```python
from build123d import *

# Parameters (mm, degrees)
CROQUIS1_R              = 1.7
SALIENTE_EXTRUIR1_DEPTH = 2
SALIENTE_EXTRUIR2_DEPTH = 6.5
MATRIZL1_COUNT          = 6
MATRIZL1_PITCH          = 2


with BuildPart() as part:
    # Croquis1 → Saliente-Extruir1 (new body)
    with BuildSketch(Plane(origin=(0, 0, 0), x_dir=(1, 0, 0), z_dir=(0, 1, 0))):
        with BuildLine():
            Line((-8, 6), (8, 6))
            Line((8, 6), (8, 3.665719575))
            ThreePointArc((8, 3.665719575), (8.133788189, 2.858848044), (8.520833333, 2.138336419))
            ThreePointArc((8.520833333, 2.138336419), (9.25, 0), (8.520833333, -2.138336419))
            ThreePointArc((8.520833333, -2.138336419), (8.133788189, -2.858848044), (8, -3.665719575))
            Line((8, -3.665719575), (8, -6))
            Line((8, -6), (-8, -6))
            Line((-8, -6), (-8, -3.665719575))
            ThreePointArc((-8, -3.665719575), (-8.133788189, -2.858848044), (-8.520833333, -2.138336419))
            ThreePointArc((-8.520833333, -2.138336419), (-9.25, 0), (-8.520833333, 2.138336419))
            ThreePointArc((-8.520833333, 2.138336419), (-8.133788189, 2.858848044), (-8, 3.665719575))
            Line((-8, 3.665719575), (-8, 6))
        make_face()
        with Locations((5.75, 0)):
            Circle(CROQUIS1_R, mode=Mode.SUBTRACT)
        with Locations((-5.75, 0)):
            Circle(CROQUIS1_R, mode=Mode.SUBTRACT)
    extrude(amount=SALIENTE_EXTRUIR1_DEPTH)

    # Croquis4 → Saliente-Extruir2 (add)
    with BuildSketch(Plane(origin=(3.25, 0, 0), x_dir=(0, 0, -1), z_dir=(1, 0, 0))):
        Polygon((-6, 2), (-4, 2), (-4.9, 2.9), (-5.1, 2.9), align=None)
    saliente_extruir2 = extrude(amount=-SALIENTE_EXTRUIR2_DEPTH)

    # MatrizL1: Saliente-Extruir2 ×6
    with Locations(*[(0, 0, -i * MATRIZL1_PITCH) for i in range(1, MATRIZL1_COUNT)]):
        add(saliente_extruir2)


solid = part.part
```
Input: part model. Units: mm. Frame: model coordinates. A direction names the side the tool comes from. Give positions to 0.01 mm unless a question says otherwise; leave off trailing zeros. Order: outer loops, then holes, each group sorted by start corner. A loop starts at its lowest first (then second) coordinate and runs counter-clockwise, first axis right, second up.
1. Cut plane D-D (x = -1). Return loops of the section in (y, z).
Computed:
outline: (0, -6) - (2, -6) - (2.9, -5.1) - (2.9, -4.9) - (2, -4) - (2.9, -3.1) - (2.9, -2.9) - (2, -2) - (2.9, -1.1) - (2.9, -0.9) - (2, 0) - (2.9, 0.9) - (2.9, 1.1) - (2, 2) - (2.9, 2.9) - (2.9, 3.1) - (2, 4) - (2.9, 4.9) - (2.9, 5.1) - (2, 6) - (0, 6) - close
2. Cut plane A-A (y = 1.8). Return loops of the section in (x, z).
Computed:
outline: (-8.52, -2.14) arc R2.5 cw to (-8, -3.67) - (-8, -6) - (8, -6) - (8, -3.67) arc R2.5 cw to (8.52, -2.14) arc R3.5 ccw to (8.52, 2.14) arc R2.5 cw to (8, 3.67) - (8, 6) - (-8, 6) - (-8, 3.67) arc R2.5 cw to (-8.52, 2.14) arc R3.5 ccw to start; hole circle Ø3.4 at (-5.75, 0); hole circle Ø3.4 at (5.75, 0)
3. Pin query (flat end, axial travel): pin 1 Ø3 at (x, z) = (-6, 2) entering from +Y; pin 2 Ø1 at (y, z) = (0.5, -4.5) entering from +X; pin 3 Ø2.5 at (x, z) = (5.75, 0) entering from -Y; pin 4 Ø0.7 at (y, z) = (2.5, -0.5) entering from -X. Return the tip coordinate at first contact, or that it passes through.
Computed:
pin 1: stops at y = 2
pin 2: stops at x = 8
pin 3: passes through
pin 4: stops at x = -3.25
4. Set-up query: faces 1 (the face through (3.25, 2.4, -1)), 2 (the face through (-3.25, 2.4, -1)), 3 (the face through (-8, 1, 5)). Return all of +Z, -Z, +X, -X, +Y, -Y with unobstructed straight access to the full face (end or side cutting, diameter ignored); none if empty.
Computed:
face 1: +Z, -Z, +X, +Y
face 2: +Z, -Z, -X, +Y
face 3: +Z, -X, +Y, -Y
5. Cut plane B-B (x = -5.75). Return loops of the section in (y, z).
Computed:
outline: (0, -6) - (2, -6) - (2, -1.7) - (0, -1.7) - close; (0, 1.7) - (2, 1.7) - (2, 6) - (0, 6) - close
6. Draft query along Z for faces 4 (the face through (0, 2.4, 0.4)), 5 (the face through (9.25, 0.99, -0.03)), 6 (the face through (3.25, 2.4, 1)), 7 (the face through (0, 2.4, -1.6)). Return one class per face: released by +Z, released by -Z, zero draft, split by the parting line, or undercut.
Computed:
face 4: undercut
face 5: split by the parting line
face 6: zero draft
face 7: undercut
7. Cut plane C-C (z = -1.5). Return loops of the section in (x, y), and give its area (3 significant figures).
Computed:
outline: (-8.91, 0) - (-6.55, 0) - (-6.55, 2) - (-8.91, 2) - close; (-4.95, 0) - (4.95, 0) - (4.95, 2) - (3.25, 2) - (3.25, 2.5) - (-3.25, 2.5) - (-3.25, 2) - (-4.95, 2) - close; (6.55, 0) - (8.91, 0) - (8.91, 2) - (6.55, 2) - close
area: 32.5 mm2
8. Line query: probe 1 along Z at (x, y) = (-5.75, 0.8); probe 2 along Z at (x, y) = (2.75, 2.4); probe 3 along Y at (x, z) = (7.5, 4.75). Output: solid intervals per line, ascending.
Computed:
probe 1: z = -6 to -1.7, 1.7 to 6
probe 2: z = -5.6 to -4.4, -3.6 to -2.4, -1.6 to -0.4, 0.4 to 1.6, 2.4 to 3.6, 4.4 to 5.6
probe 3: y = 0 to 2
